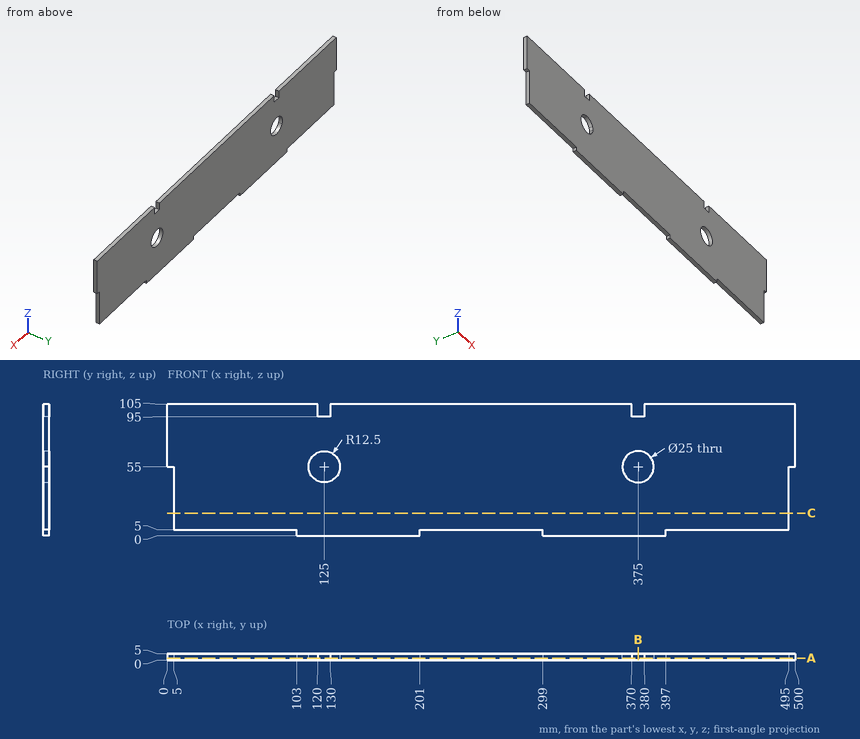
The drawing under review shows one solid part. Ordinate dimensions are in mm from its lowest x, y, z. Coordinates: 2 decimals unless noted, no trailing zeros. Write each loop counter-clockwise with the first axis right and the second up, starting at its lowest first coordinate (ties: lowest second). Pieces come first, ordered by that corner, then holes. Notation, with made-up numbers: (59, 4.5) -> (79, 4.5) arc R16 ccw to (79, 32.5) -> close; hole circle Ø2 at (-7.5, 88.5). An arc over 180 degrees is marked (long way). Write each question's results on one line, items separated by ' | '. Start each with the question number.
1) Consider section A-A (y = 1.5). Write out the cut boundary in (x, z).
2) Consider section C-C (z = 18). Write out the cut boundary in (x, y), plus the area to 3 significant figures.
3) Consider section B-B (x = 375). Write out the cut boundary in (y, z).
4) Insertion check: pin 1 (2.5 mm diameter, centred on x = 239, y = 3.5, fed in from -Z); pin 2 (2.5 mm diameter, centred on y = 2, z = 3, fed in from +X). Each pin has a flat end and moves straight along its axis. Give the tip position at first contact, or say it passes through.
5) Wall thickness on L1, parallel to Z at x = 375, y = 3.5; L2, parallel to X at y = 3.5, z = 50; L3, parallel to Z at x = 221.5, y = 0.7: over which ranges is each line inside the solid? List them lowest first. Write a range as [from, to].
Geometry says:
1) outline: (0, 55) -> (5, 55) -> (5, 5) -> (103, 5) -> (103, 0) -> (201, 0) -> (201, 5) -> (299, 5) -> (299, 0) -> (397, 0) -> (397, 5) -> (495, 5) -> (495, 55) -> (500, 55) -> (500, 105) -> (380, 105) -> (380, 95) -> (370, 95) -> (370, 105) -> (130, 105) -> (130, 95) -> (120, 95) -> (120, 105) -> (0, 105) -> close; hole circle Ø25 at (125, 55); hole circle Ø25 at (375, 55)
2) outline: (5, 0) -> (495, 0) -> (495, 5) -> (5, 5) -> close | area: 2,450 mm^2
3) outline: (0, 0) -> (5, 0) -> (5, 42.5) -> (0, 42.5) -> close; (0, 67.5) -> (5, 67.5) -> (5, 95) -> (0, 95) -> close
4) pin 1: z = 5 | pin 2: x = 397
5) L1: [0, 42.5], [67.5, 95] | L2: [5, 113.54], [136.46, 363.54], [386.46, 495] | L3: [5, 105]
